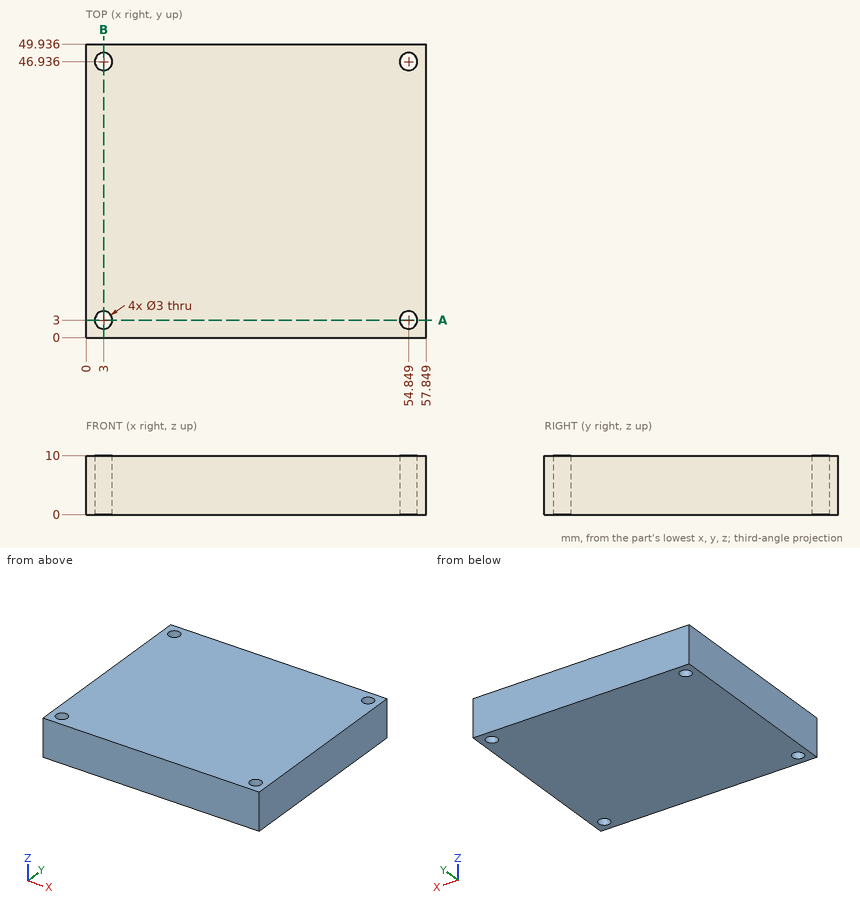
Could you check a few things on this drawing? It's one solid part, dimensions in mm from its lowest x, y, z. Give positions to 0.01 mm unless a question says otherwise; leave off trailing zeros. Order: outer loops, then holes, each group sorted by start corner. A loop starts at its lowest first (then second) coordinate and runs counter-clockwise, first axis right, second up.
1. Suppose I cut it at B-B (x = 3). Write out the boundary of the cut face in (y, z), plus the area to 3 significant figures.
Answers below:
outline: (0, 0) - (1.5, 0) - (1.5, 10) - (0, 10) - close; (4.5, 0) - (45.44, 0) - (45.44, 10) - (4.5, 10) - close; (48.44, 0) - (49.94, 0) - (49.94, 10) - (48.44, 10) - close
area: 439 mm2
2. I need wall thicknesses on L1, parallel to Y at x = 3, z = 3; L2, parallel to Y at x = 3.5, z = 5. Which ranges of each line are inside material? Lowest first, please.
Answers below:
L1: y = 0 to 1.5, 4.5 to 45.44, 48.44 to 49.94
L2: y = 0 to 1.59, 4.41 to 45.52, 48.35 to 49.94
3. Suppose I cut it at A-A (y = 3). Write out the boundary of the cut face in (x, z), plus the area to 3 significant figures.
Answers below:
outline: (0, 0) - (1.5, 0) - (1.5, 10) - (0, 10) - close; (4.5, 0) - (53.35, 0) - (53.35, 10) - (4.5, 10) - close; (56.35, 0) - (57.85, 0) - (57.85, 10) - (56.35, 10) - close
area: 518 mm2
